from build123d import *

# Parameters (mm, degrees)
SKETCH1_R           = 32.5
SKETCH1_R_2         = 12.7
SKETCH1_R_3         = 1.65
BOSS_EXTRUDE1_DEPTH = 5.842
SKETCH2_R           = 1.5
CUT_EXTRUDE2_DEPTH  = 47.331727401


with BuildPart() as part:
    # Sketch1 → Boss-Extrude1 (new body)
    with BuildSketch(Plane.XY):
        Circle(SKETCH1_R)
        Circle(SKETCH1_R_2, mode=Mode.SUBTRACT)
        with Locations((22, 0)):
            Circle(SKETCH1_R_3, mode=Mode.SUBTRACT)
        with Locations((0, -22)):
            Circle(SKETCH1_R_3, mode=Mode.SUBTRACT)
        with Locations((-22, 0)):
            Circle(SKETCH1_R_3, mode=Mode.SUBTRACT)
    extrude(amount=BOSS_EXTRUDE1_DEPTH)

    # Sketch2 → Cut-Extrude2 (cut, through all)
    with BuildSketch(Plane.XY.offset(5.842)):
        with Locations((-15.556349186, -15.556349186)):
            Circle(SKETCH2_R)
        with Locations((-15.556349186, 15.556349186)):
            Circle(SKETCH2_R)
        with Locations((15.556349186, 15.556349186)):
            Circle(SKETCH2_R)
        with Locations((15.556349186, -15.556349186)):
            Circle(SKETCH2_R)
    extrude(amount=-CUT_EXTRUDE2_DEPTH, mode=Mode.SUBTRACT)


solid = part.part
The model under review builds one solid part; all positions refer to its coordinate system, in mm. Give positions to 0.01 mm unless a question says otherwise; leave off trailing zeros. Loops run counter-clockwise (first coordinate to the right, second up) from the corner with the lowest first, then second, coordinate; pieces in that order, holes last. Notation, with made-up numbers: (-37, 74.5) -> (8, 74.5) arc R31 cw to (8, 111.5) -> close; hole circle Ø6 at (19, 81.5). An arc over 180 degrees is marked (long way). Answer as a JSON object with one key per item and string values. Group by question number.
Q1. Take a section at C-C (x = 22). Write out the cut boundary in (y, z).
Q2. Take a section at B-B (y = 0). Write out the cut boundary in (x, z).
Q3. Draft analysis for pull direction X (two halves, no side actions). For faces 1 (the flat face through (14, 0, 0)), 2 (the cylindrical face through (31, 9.76, 2.88)), 3 (the cylindrical face through (-14.75, 16.82, 2.96)), 4 (the cylindrical face through (14.45, 16.57, 2.96)), state which applies: pulls with the +X half, pulls with the -X half, needs draft (parallel to the pull), parting line crosses it, or undercut.
Q4. Take a section at A-A (x = 0). Write out the cut boundary in (y, z).
Q5. Wall thickness on line 1 along Y through (x, z) = (0, 3.4); line 2 along Y through (x, z) = (-1, 0.4); line 3 along X through (y, z) = (16, 3.9): over which ranges is each line inside the solid? List them lowest first.
Q6. Insertion check: pin 1 (2.5 mm diameter, centred on x = -15.56, y = -15.56, fed in from -Z); pin 2 (2 mm diameter, centred on y = 12, z = 3, fed in from +X); pin 3 (1.5 mm diameter, centred on x = 10, z = 3, fed in from -Y). Each pin has a flat end and moves straight along its axis. Give the tip position at first contact, or say it passes through.
Answer below:
{
 "1": {"outline": "(-23.92, 0) -> (-1.65, 0) -> (-1.65, 5.84) -> (-23.92, 5.84) -> close; (1.65, 0) -> (23.92, 0) -> (23.92, 5.84) -> (1.65, 5.84) -> close"},
 "2": {"outline": "(-32.5, 0) -> (-23.65, 0) -> (-23.65, 5.84) -> (-32.5, 5.84) -> close; (-20.35, 0) -> (-12.7, 0) -> (-12.7, 5.84) -> (-20.35, 5.84) -> close; (12.7, 0) -> (20.35, 0) -> (20.35, 5.84) -> (12.7, 5.84) -> close; (23.65, 0) -> (32.5, 0) -> (32.5, 5.84) -> (23.65, 5.84) -> close"},
 "3": {"face 1": "needs draft", "face 2": "parting line crosses it", "face 3": "undercut", "face 4": "undercut"},
 "4": {"outline": "(-32.5, 0) -> (-23.65, 0) -> (-23.65, 5.84) -> (-32.5, 5.84) -> close; (-20.35, 0) -> (-12.7, 0) -> (-12.7, 5.84) -> (-20.35, 5.84) -> close; (12.7, 0) -> (32.5, 0) -> (32.5, 5.84) -> (12.7, 5.84) -> close"},
 "5": {"line 1": "y = -32.5 to -23.65, -20.35 to -12.7, 12.7 to 32.5", "line 2": "y = -32.48 to -23.31, -20.69 to -12.66, 12.66 to 32.48", "line 3": "x = -28.29 to -16.99, -14.12 to 14.12, 16.99 to 28.29"},
 "6": {"pin 1": "passes through", "pin 2": "stops at x = 30.58", "pin 3": "stops at y = -31.16"}
}
